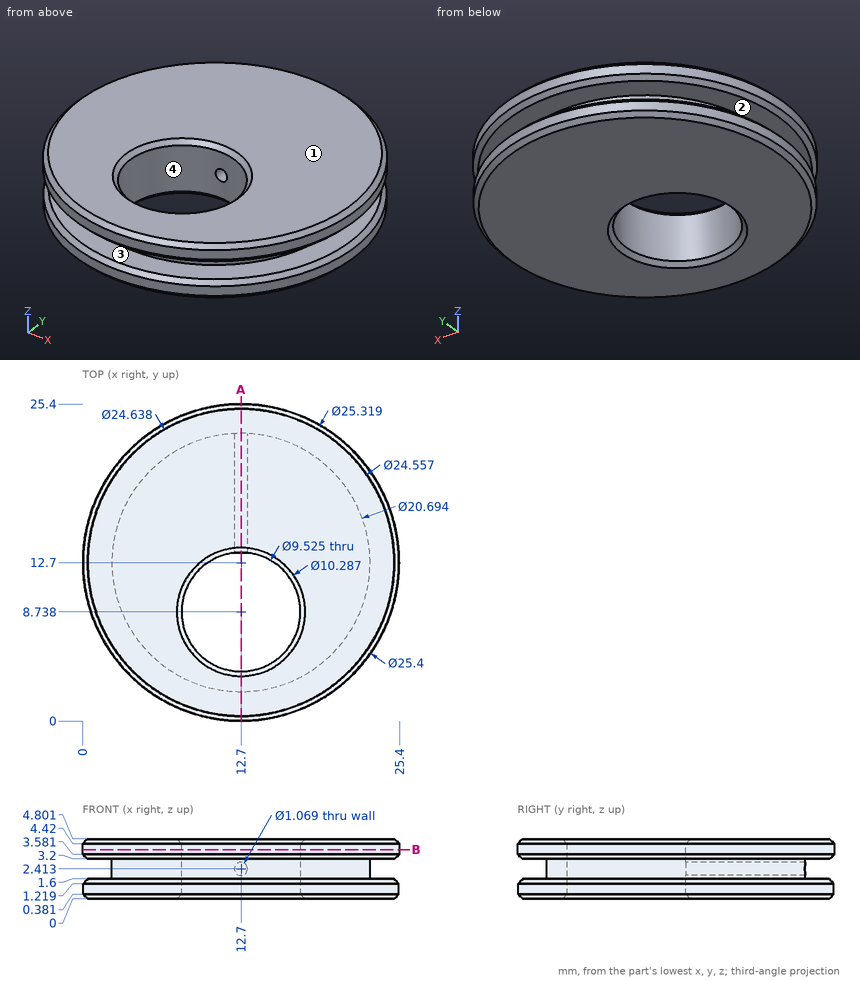
Print and shaded views of the part. All mm, measured from the part's lowest x, y and z. A direction names the side the tool comes from. Round coordinates to 2 decimals unless told otherwise and drop trailing zeros. Write each loop counter-clockwise with the first axis right and the second up, starting at its lowest first coordinate (ties: lowest second). Pieces come first, ordered by that corner, then holes. Notation, with made-up numbers: M -21,61 L 34,61 A15 ccw 34,78 Z; hole C 30,8 d8. An arc over 180 degrees is marked long. Use a Markdown table: item, result. Add a question column.
1. Flat gauge pins, fed straight in: P1, Ø3, axis at x = 4, y = 20.5, coming from the -Z side; P2, Ø1, axis at x = 12.7, z = 2.41, coming from the -Y side; P3, Ø1, axis at x = 19, z = 1, coming from the +Y side; P4, Ø1, axis at y = 10.5, z = 1, coming from the +X side (1 decimal). Where does each tip first touch, or does it go through?
2. Slice it at B-B on z = 3.95. Give the cut face in (x, y) (1 decimal).
3. Drill centre lines: probe 1 along Z at (x, y) = (12.7, 15.5); probe 2 along Z at (x, y) = (13.5, 23.75); probe 3 along X at (y, z) = (21.25, 2.1) (1 decimal). Where is each one in solid material? Low to high.
4. Slice it at A-A on x = 12.7. Give the number of separate pieces and of enclosed holes in the cut face.
5. 3-axis set-ups, long thin cutter, end or side, ignore diameter. For the marked faces 1 and 2: which of +Z, -Z, +X, -X, +Y, -Y reach the whole face in a straight line?
6. Pull direction X, two halves, no side cores. Call the marked faces 3 and 4: released by +X, released by -X, zero draft, split by the parting line, or undercut.
Reply:
| question | item | result |
|---|---|---|
| 1 | P1 | stops at z = 0 |
| 1 | P2 | stops at y = 2.35 |
| 1 | P3 | stops at y = 23.95 |
| 1 | P4 | stops at x = 25.2 |
| 2 | outline | C 12.7,12.7 d25.4; hole C 12.7,8.7 d9.5 |
| 3 | probe 1 | z = 0 to 1.88, 2.95 to 4.8 |
| 3 | probe 2 | z = 0 to 1.6, 3.2 to 4.8 |
| 3 | probe 3 | x = 6.9 to 12.3, 13.1 to 18.5 |
| 4 | separate pieces | 3 |
| 4 | enclosed holes | 0 |
| 5 | face 1 | +Z, +X, -X, +Y, -Y |
| 5 | face 2 | none |
| 6 | face 3 | zero draft |
| 6 | face 4 | undercut |
